CAD build for the part. Positions are in the model's coordinates, mm. Face numbers are marked on the shaded views. A direction names the side the tool comes from. Round coordinates to 2 decimals unless told otherwise and drop trailing zeros. Write each loop counter-clockwise with the first axis right and the second up, starting at its lowest first coordinate (ties: lowest second). Pieces come first, ordered by that corner, then holes. Notation, with made-up numbers: M -39.75,-26 L -4.75,-26 A30 cw -4.75,2 Z; hole C -18.75,65 d1. An arc over 180 degrees is marked long. Write each question's results on one line, items separated by ' | '. Start each with the question number.
```python
from build123d import *

# Parameters (mm, degrees)
BOSS_EXTRUDE1_DEPTH = 15
SKETCH2_R           = 1.5
CUT_EXTRUDE1_DEPTH  = 32.171300903
CHAMFER1_SIZE       = 0.5


with BuildPart() as part:
    # Sketch1 → Boss-Extrude1 (new, symmetric)
    with BuildSketch(Plane.XY):
        with BuildLine():
            Line((-15, 13.1), (-15, 2.04))
            Line((-15, 2.04), (15, 2.04))
            Line((15, 2.04), (15, 13.1))
            Line((15, 13.1), (23.7, 13.1))
            Line((23.7, 13.1), (23.7, 11.6))
            Line((23.7, 11.6), (16.55, 11.6))
            Line((16.55, 11.6), (16.55, 9.4))
            Line((16.55, 9.4), (23.7, 9.4))
            Line((23.7, 9.4), (23.7, 7.9))
            Line((23.7, 7.9), (16.55, 7.9))
            Line((16.55, 7.9), (16.55, 5.09))
            Line((16.55, 5.09), (23.7, 5.09))
            Line((23.7, 5.09), (23.7, 3.59))
            Line((23.7, 3.59), (19.35, 3.59))
            Line((19.35, 3.59), (18.254412307, 3.294047964))
            ThreePointArc((18.254412307, 3.294047964), (17.7, 2.57), (18.254412307, 1.845952036))
            Line((18.254412307, 1.845952036), (19.35, 1.55))
            Line((19.35, 1.55), (23.7, 1.55))
            Line((23.7, 1.55), (23.7, 0))
            Line((23.7, 0), (16.5, 0))
            Line((16.5, 0), (16.5, -0.5))
            Line((16.5, -0.5), (-16.5, -0.5))
            Line((-16.5, -0.5), (-16.5, 0))
            Line((-16.5, 0), (-23.7, 0))
            Line((-23.7, 0), (-23.7, 1.55))
            Line((-23.7, 1.55), (-19.35, 1.55))
            Line((-19.35, 1.55), (-18.254412307, 1.845952036))
            ThreePointArc((-18.254412307, 1.845952036), (-17.7, 2.57), (-18.254412307, 3.294047964))
            Line((-18.254412307, 3.294047964), (-19.35, 3.59))
            Line((-19.35, 3.59), (-23.7, 3.59))
            Line((-23.7, 3.59), (-23.7, 5.09))
            Line((-23.7, 5.09), (-16.55, 5.09))
            Line((-16.55, 5.09), (-16.55, 7.9))
            Line((-16.55, 7.9), (-23.7, 7.9))
            Line((-23.7, 7.9), (-23.7, 9.4))
            Line((-23.7, 9.4), (-16.55, 9.4))
            Line((-16.55, 9.4), (-16.55, 11.6))
            Line((-16.55, 11.6), (-23.7, 11.6))
            Line((-23.7, 11.6), (-23.7, 13.1))
            Line((-23.7, 13.1), (-15, 13.1))
        make_face()
    extrude(amount=BOSS_EXTRUDE1_DEPTH, both=True)

    # Sketch2 → Cut-Extrude1 (cut, through all)
    with BuildSketch(Plane.XZ.offset(0.5)):
        with Locations(Location((0, 4.65, 0), (0, 0, 270))):
            Circle(SKETCH2_R)
    extrude(amount=-CUT_EXTRUDE1_DEPTH, mode=Mode.SUBTRACT)

    # Chamfer1
    chamfer1_edges = [part.edges().sort_by_distance(p)[0] for p in [
        (0, -0.5, 6.15),
    ]]
    chamfer(chamfer1_edges, length=CHAMFER1_SIZE)


solid = part.part
```
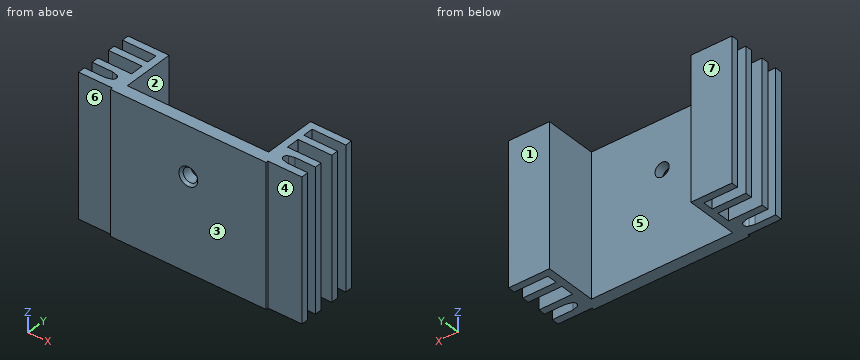
1) 3-axis set-ups, long thin cutter, end or side, ignore diameter. For the marked faces 3, 4, 5, 6 and 7: which of +Z, -Z, +X, -X, +Y, -Y reach the whole face in a straight line?
2) Wall check: line 1 along X through (y, z) = (1.2, 4.65); line 2 along Y through (x, z) = (-20.5, 7); line 3 along X through (y, z) = (9, -4.75). Give the ranges that are in metal, low to high. Write a range as from..to.
3) Drop flat-ended pins along their axis: pin 1 Ø5 at (x, z) = (-7.5, -9) entering from +Y; pin 2 Ø3.5 at (x, z) = (-21.5, 4.5) entering from -Y; pin 3 Ø1.4 at (y, z) = (6, -2) entering from +X. Give the stop position or say it passes through.
4) Pull direction X, two halves, no side cores. Call the marked faces 1 and 2: pulls with the +X half, pulls with the -X half, needs draft (parallel to the pull), parting line crosses it, or undercut.
5) Saw through at B-B, the plane y = 8.5. Write the cut outline in (x, z).
6) Saw through at A-A, the plane x = 0. Write the cut outline in (y, z).
7) Saw through at C-C, the plane x = -6. Write the cut outline in (y, z), plus the area to 3 significant figures.
Filled sheet:
1) face 3: +Z, -Z, +X, -X, -Y | face 4: +Z, -Z, +X, -Y | face 5: +Z, -Z, +Y | face 6: +Z, -Z, -X, -Y | face 7: +Z, -Z, +X, -X, +Y
2) line 1: x = -23.7..-1.5, 1.5..23.7 | line 2: y = 0..1.55, 3.59..5.09, 7.9..9.4, 11.6..13.1 | line 3: x = -23.7..-15, 15..23.7
3) pin 1: stops at y = 2.04 | pin 2: stops at y = 0 | pin 3: stops at x = 16.55
4) face 1: needs draft | face 2: undercut
5) outline: M -23.7,-15 L -15,-15 L -15,15 L -23.7,15 Z; M 15,-15 L 23.7,-15 L 23.7,15 L 15,15 Z
6) outline: M -0.5,-15 L 2.04,-15 L 2.04,3.15 L 0,3.15 L -0.5,2.65 Z; M -0.5,6.65 L 0,6.15 L 2.04,6.15 L 2.04,15 L -0.5,15 Z
7) outline: M -0.5,-15 L 2.04,-15 L 2.04,15 L -0.5,15 Z | area: 76.2 mm^2
